Source: CAD feature listing. Evaluate the final solid. Frame: model axes, mm. A direction names the side the tool comes from. Give positions to 0.01 mm unless a question says otherwise; leave off trailing zeros. Loops run counter-clockwise (first coordinate to the right, second up) from the corner with the lowest first, then second, coordinate; pieces in that order, holes last. Notation, with made-up numbers: (62.5, -14) -> (121.5, -14) arc R26 cw to (121.5, 5) -> close; hole circle Ø8 at (70.25, 11.5). An arc over 180 degrees is marked (long way). Answer as a JSON object with one key per item and string values. Group by question number.
from build123d import *

# Parameters (mm, degrees)
EXTRUDE_1_DEPTH      = 3
EXTRUDE_1_DEPTH_BACK = 3
FILLET_1_R           = 0.5
SKETCH_3_W           = 5.9
SKETCH_3_H           = 0.8
CUT_EXTRUDE_1_DEPTH  = 0.5
SKETCH_4_W           = 5
SKETCH_4_H           = 0.5
CUT_EXTRUDE_2_DEPTH  = 0.5
SKETCH_5_W           = 2.75
SKETCH_5_H           = 5.4
CUT_EXTRUDE_3_DEPTH  = 0.2
SKETCH_6_R           = 0.35
EXTRUDE_3_DEPTH      = 0.2
SKETCH_2_W           = 0.4
SKETCH_2_H           = 0.4
EXTRUDE_2_DEPTH      = 2.5


with BuildPart() as part:
    # Эскиз1 → Бобышка-Вытянуть1 (new, two sides: drawn at the far end of the back side and taken through both)
    with BuildSketch(Plane(origin=(0, 0, 0), x_dir=(1, 0, 0), z_dir=(0, 1, 0)).offset(-EXTRUDE_1_DEPTH_BACK)):
        Polygon((6.5, 0), (-6.5, 0), (-6.5, -10), (-2.5, -10), (-2.5, -2), (2.5, -2), (2.5, -10), (6.5, -10), align=None)
    extrude(amount=EXTRUDE_1_DEPTH + EXTRUDE_1_DEPTH_BACK)

    # Скругление1
    fillet_1_edges = [part.edges().sort_by_distance(p)[0] for p in [
        (2.5, 0, 10),
        (-2.5, 0, 10),
    ]]
    fillet(fillet_1_edges, radius=FILLET_1_R)

    # Эскиз3 → Вырез-Вытянуть1 (cut)
    with BuildSketch(Plane(origin=(6.5, 0, 0), x_dir=(0, 0, -1), z_dir=(1, 0, 0))):
        with Locations((-7.05, 0)):
            Rectangle(SKETCH_3_W, SKETCH_3_H)
    cut_extrude_1 = extrude(amount=-CUT_EXTRUDE_1_DEPTH, mode=Mode.SUBTRACT)

    # Эскиз4 → Вырез-Вытянуть2 (cut)
    with BuildSketch(Plane.ZY.offset(-2.5)):
        with Locations((4.5, 0)):
            Rectangle(SKETCH_4_W, SKETCH_4_H)
    cut_extrude_2 = extrude(amount=-CUT_EXTRUDE_2_DEPTH, mode=Mode.SUBTRACT)

    # Зеркальное отражение1: Вырез-Вытянуть1, Вырез-Вытянуть2 across plane
    add(cut_extrude_1.mirror(Plane(origin=(0, 0, 0), x_dir=(0, 0, 1), z_dir=(1, 0, 0))), mode=Mode.SUBTRACT)
    add(cut_extrude_2.mirror(Plane(origin=(0, 0, 0), x_dir=(0, 0, 1), z_dir=(1, 0, 0))), mode=Mode.SUBTRACT)

    # Эскиз5 → Вырез-Вытянуть3 (cut)
    with BuildSketch(Plane.XY.offset(10)):
        with Locations((-4.625, 0)):
            Rectangle(SKETCH_5_W, SKETCH_5_H)
        with Locations((4.625, 0)):
            Rectangle(SKETCH_5_W, SKETCH_5_H)
    extrude(amount=-CUT_EXTRUDE_3_DEPTH, mode=Mode.SUBTRACT)

    # Эскиз6 → Бобышка-Вытянуть3 (add)
    with BuildSketch(Plane.XY.offset(9.8)):
        with Locations(Location((-4.625, 2, 0), (0, 0, 180))):
            Circle(SKETCH_6_R)
        Polygon((4.725, -2), (4.725, -0.7), (5.475, -0.7), (4.725, 0.5), (5.475, 0.5), (5.475, 0.7), (4.725, 0.7), (4.725, 2), (4.525, 2), (4.525, 0.7), (3.775, 0.7), (3.775, 0.5), (4.525, 0.5), (3.775, -0.7), (4.525, -0.7), (4.525, -2), align=None)
    extrude(amount=EXTRUDE_3_DEPTH)

    # Эскиз2 → Бобышка-Вытянуть2 (add)
    with BuildSketch(Plane(origin=(0, 0, 0), x_dir=(-1, 0, 0), z_dir=(0, 0, -1))):
        with Locations((5, 1.27)):
            Rectangle(SKETCH_2_W, SKETCH_2_H)
        with Locations((-5, 1.27)):
            Rectangle(SKETCH_2_W, SKETCH_2_H)
        with Locations((5, -1.27)):
            Rectangle(SKETCH_2_W, SKETCH_2_H)
        with Locations((-5, -1.27)):
            Rectangle(SKETCH_2_W, SKETCH_2_H)
    extrude(amount=EXTRUDE_2_DEPTH)


solid = part.part
(1) Section query B-B on y = -1.7. Return the cut outline in (x, z) (3 decimals).
(2) Material intervals for line 1 (X direction, y = 0.35, z = 6.25); line 2 (Y direction, x = 2.75, z = 3.5); line 3 (X direction, y = -0.9, z = 3), sorted ascending. Write a range as from..to.
(3) Section query A-A on z = 3.5. Return the cut outline in (x, y), plus the area to 3 significant figures.
(4) Mould query, pull axis X, two halves, no side actions, for faces 1 (the face through (6.2, 0.7, 10)), 2 (the face through (0, 0, 2)), 3 (the face through (-6.5, -1, 5)). Classes: pulls with the +X half, pulls with the -X half, needs draft (parallel to the pull), parting line crosses it, or undercut.
(5) First-contact query: pin 1 (1.5 mm diameter, centred on x = 4, y = 0, fed in from -Z). Flat tip, straight axial feed; report the tip coordinate or a pass-through.
(6) Access query for faces 4 (the face through (-3, -3, 5)), 5 (the face through (-2.5, -1, 6)), 6 (the face through (-5, 0, 9.8)). Directions: +Z, -Z, +X, -X, +Y, -Y. A direction counts if a zero-diameter tool reaches every point of the face in a straight line with its end or side. Return the directions, or none.
(7) Section query C-C on z = 8. Return the cut outline in (x, y).
Result:
{
 "1": {"outline": "(-6.5, 0) -> (6.5, 0) -> (6.5, 10) -> (6, 10) -> (6, 9.8) -> (4.725, 9.8) -> (4.725, 10) -> (4.525, 10) -> (4.525, 9.8) -> (3.25, 9.8) -> (3.25, 10) -> (3, 10) arc R0.5 ccw to (2.5, 9.5) -> (2.5, 2) -> (-2.5, 2) -> (-2.5, 9.5) arc R0.5 ccw to (-3, 10) -> (-3.25, 10) -> (-3.25, 9.8) -> (-6, 9.8) -> (-6, 10) -> (-6.5, 10) -> close"},
 "2": {"line 1": "-6..-2.5, 2.5..6", "line 2": "-3..-0.25, 0.25..3", "line 3": "-6.5..-2.5, 2.5..6.5"},
 "3": {"outline": "(-6.5, -3) -> (-2.5, -3) -> (-2.5, -0.25) -> (-3, -0.25) -> (-3, 0.25) -> (-2.5, 0.25) -> (-2.5, 3) -> (-6.5, 3) -> close; (2.5, -3) -> (6.5, -3) -> (6.5, 3) -> (2.5, 3) -> (2.5, 0.25) -> (3, 0.25) -> (3, -0.25) -> (2.5, -0.25) -> close", "area": "47.5 mm²"},
 "4": {"face 1": "needs draft", "face 2": "undercut", "face 3": "pulls with the -X half"},
 "5": {"pin 1": "z = 0"},
 "6": {"face 4": "+Z, -Z, +X, -X, -Y", "face 5": "+Z, +Y, -Y", "face 6": "+Z"},
 "7": {"outline": "(-6.5, -3) -> (-2.5, -3) -> (-2.5, 3) -> (-6.5, 3) -> (-6.5, 0.4) -> (-6, 0.4) -> (-6, -0.4) -> (-6.5, -0.4) -> close; (2.5, -3) -> (6.5, -3) -> (6.5, -0.4) -> (6, -0.4) -> (6, 0.4) -> (6.5, 0.4) -> (6.5, 3) -> (2.5, 3) -> close"}
}
